Autodesk Inventor part; units mm, degrees
ref_plane "YZ Plane" through (0, 0, 0) normal (1, 0, 0) x (0, 1, 0)
ref_plane "XZ Plane" through (0, 0, 0) normal (0, 1, 0) x (-1, 0, 0)
ref_plane "XY Plane" through (0, 0, 0) normal (0, 0, 1) x (1, 0, 0)
sketch "Sketch1" plane through (0, 0, 0) normal (0, 1, 0) x (-1, 0, 0)
  circle A0 centre (0, 0) radius 2.4765
  circle A1 centre (-8.1903, -11.4773) radius 6 construction
  circle A2 centre (0, -14.1) radius 6 construction
  line L0 (0, -14.1) -> (-8.1903, -11.4773) construction
  circle A3 centre (-8.1903, -11.4773) radius 5.3 construction
  circle A4 centre (0, -14.1) radius 5.3 construction
  line L1 (-4.7712, -16.4078) -> (-5.6471, -16.1273)
  circle A5 centre (0, 0) radius 12.5 construction
  line L2 (-8.1903, -11.4773) -> (0, 0) construction
  arc A6 (-4.7712, -16.4078) -> (-2.2465, -12.2965) centre (-8.1903, -11.4773) ccw
  arc A7 (-5.3141, -11.3142) -> (-5.6471, -16.1273) centre (0, -14.1) ccw
  line L3 (2.3149, -16.9299) -> (1.4006, -17.0299)
  arc A8 (2.3149, -16.9299) -> (2.9491, -12.1471) centre (-2.814, -13.8163) ccw
  arc A9 (-0.2527, -12.4974) -> (1.4006, -17.0299) centre (5.735, -12.881) ccw
  line L4 (9.0008, -14.5246) -> (8.2062, -14.9879)
  arc A10 (9.0008, -14.5246) -> (7.6348, -9.8974) centre (3.0489, -13.7664) ccw
  arc A11 (4.8523, -11.5198) -> (8.2062, -14.9879) centre (10.4783, -9.4347) ccw
  line L5 (14.1303, -9.6079) -> (13.5929, -10.3543)
  arc A12 (14.1303, -9.6079) -> (11.0004, -5.9364) centre (8.3846, -11.3361) ccw
  arc A13 (9.1183, -8.5502) -> (13.5929, -10.3543) centre (13.4099, -4.3571) ccw
  line L6 (16.8166, -3.03) -> (16.6292, -3.9304)
  arc A14 (16.8166, -3.03) -> (12.4639, -0.9489) centre (12.2706, -6.9458) ccw
  arc A15 (11.8077, -4.1023) -> (16.6292, -3.9304) centre (14.0228, 1.4739) ccw
  line L7 (16.5951, 4.0719) -> (16.7902, 3.1731)
  arc A16 (16.5951, 4.0719) -> (11.7723, 4.2027) centre (14.0348, -1.3544) ccw
  arc A17 (12.4554, 1.055) -> (16.7902, 3.1731) centre (12.211, 7.05) ccw
  line L8 (13.5042, 10.4697) -> (14.048, 9.7279)
  arc A18 (13.5042, 10.4697) -> (9.0451, 8.6276) centre (13.3723, 4.4712) ccw
  arc A19 (10.9495, 6.0298) -> (14.048, 9.7279) centre (8.2878, 11.4071) ccw
  line L9 (8.0783, 15.0572) -> (8.8768, 14.6007)
  arc A20 (8.0783, 15.0572) -> (4.754, 11.5607) centre (10.3976, 9.5236) ccw
  arc A21 (7.5503, 9.9621) -> (8.8768, 14.6007) centre (2.9316, 13.7919) ccw
  line L10 (1.2556, 17.0412) -> (2.1707, 16.949)
  arc A22 (1.2556, 17.0412) -> (-0.3592, 12.4948) centre (5.6251, 12.9294) ccw
  arc A23 (2.8456, 12.1718) -> (2.1707, 16.949) centre (-2.9316, 13.7919) ccw
  line L11 (-5.7843, 16.0786) -> (-4.9107, 16.3665)
  arc A24 (-5.7843, 16.0786) -> (-5.4102, 11.2685) centre (-0.1201, 14.0995) ccw
  arc A25 (-2.3511, 12.2769) -> (-4.9107, 16.3665) centre (-8.2878, 11.4071) ccw
  line L12 (-11.824, 12.3359) -> (-11.1431, 12.9542)
  arc A26 (-11.824, 12.3359) -> (-9.5258, 8.0938) centre (-5.8445, 12.8317) ccw
  arc A27 (-7.1413, 10.2592) -> (-11.1431, 12.9542) centre (-12.211, 7.05) ccw
  line L13 (-15.8192, 6.4601) -> (-15.4486, 7.302)
  arc A28 (-15.8192, 6.4601) -> (-11.9943, 3.5195) centre (-10.5583, 9.3452) ccw
  arc A29 (-10.6967, 6.4676) -> (-15.4486, 7.302) centre (-14.0228, 1.4739) ccw
  line L14 (-17.0791, -0.5326) -> (-17.083, 0.3871)
  arc A30 (-17.0791, -0.5326) -> (-12.3888, -1.6633) centre (-13.4465, 4.2428) ccw
  arc A31 (-12.4026, 1.5577) -> (-17.083, 0.3871) centre (-13.4099, -4.3571) ccw
  line L15 (-15.3859, -7.4333) -> (-15.7636, -6.5946)
  arc A32 (-15.3859, -7.4333) -> (-10.6413, -6.5585) centre (-14.0097, -1.5932) ccw
  arc A33 (-11.9639, -3.6216) -> (-15.7636, -6.5946) centre (-10.4783, -9.4347) ccw
  arc A34 (-2.2465, -12.2965) -> (-0.2527, -12.4974) centre (0, 0) ccw
  arc A35 (2.9491, -12.1471) -> (4.8523, -11.5198) centre (0, 0) ccw
  arc A36 (7.6348, -9.8974) -> (9.1183, -8.5502) centre (0, 0) ccw
  arc A37 (11.0004, -5.9364) -> (11.8077, -4.1023) centre (0, 0) ccw
  arc A38 (12.4639, -0.9489) -> (12.4554, 1.055) centre (0, 0) ccw
  arc A39 (11.7723, 4.2027) -> (10.9495, 6.0298) centre (0, 0) ccw
  arc A40 (9.0451, 8.6276) -> (7.5503, 9.9621) centre (0, 0) ccw
  arc A41 (4.754, 11.5607) -> (2.8456, 12.1718) centre (0, 0) ccw
  arc A42 (-0.3592, 12.4948) -> (-2.3511, 12.2769) centre (0, 0) ccw
  arc A43 (-5.4102, 11.2685) -> (-7.1413, 10.2592) centre (0, 0) ccw
  arc A44 (-9.5258, 8.0938) -> (-10.6967, 6.4676) centre (0, 0) ccw
  arc A45 (-11.9943, 3.5195) -> (-12.4026, 1.5577) centre (0, 0) ccw
  arc A46 (-12.3888, -1.6633) -> (-11.9639, -3.6216) centre (0, 0) ccw
  arc A47 (-10.6413, -6.5585) -> (-9.4565, -8.1746) centre (0, 0) ccw
  line L16 (-11.0323, -13.0486) -> (-11.7185, -12.4361)
  arc A48 (-11.0323, -13.0486) -> (-7.0537, -10.3196) centre (-12.1505, -7.1537) ccw
  arc A49 (-9.4565, -8.1746) -> (-11.7185, -12.4361) centre (-5.735, -12.881) ccw
  arc A50 (-7.0537, -10.3196) -> (-5.3141, -11.3142) centre (0, 0) ccw
  point P0 (4.8523, -11.5198)
  point P1 (9.1183, -8.5502)
  point P2 (11.8077, -4.1023)
  point P3 (12.4554, 1.055)
  point P4 (10.9495, 6.0298)
  point P5 (7.5503, 9.9621)
  point P6 (2.8456, 12.1718)
  point P7 (-2.3511, 12.2769)
  point P8 (-7.1413, 10.2592)
  point P9 (-10.6967, 6.4676)
  point P10 (-12.4026, 1.5577)
  point P11 (-11.9639, -3.6216)
  point P12 (-9.4565, -8.1746)
  point P13 (-2.2465, -12.2965)
  point P14 (-0.2527, -12.4974)
  point P15 (2.9491, -12.1471)
  point P16 (4.8523, -11.5198)
  point P17 (7.6348, -9.8974)
  point P18 (9.1183, -8.5502)
  point P19 (11.0004, -5.9364)
  point P20 (11.8077, -4.1023)
  point P21 (12.4639, -0.9489)
  point P22 (12.4554, 1.055)
  point P23 (11.7723, 4.2027)
  point P24 (10.9495, 6.0298)
  point P25 (9.0451, 8.6276)
  point P26 (7.5503, 9.9621)
  point P27 (4.754, 11.5607)
  point P28 (2.8456, 12.1718)
  point P29 (-0.3592, 12.4948)
  point P30 (-2.3511, 12.2769)
  point P31 (-5.4102, 11.2685)
  point P32 (-7.1413, 10.2592)
  point P33 (-9.5258, 8.0938)
  point P34 (-10.6967, 6.4676)
  point P35 (-11.9943, 3.5195)
  point P36 (-12.4026, 1.5577)
  point P37 (-12.3888, -1.6633)
  point P38 (-11.9639, -3.6216)
  point P39 (-10.6413, -6.5585)
  point P40 (-5.3141, -11.3142)
  point P41 (-9.4565, -8.1746)
  point P42 (-7.0537, -10.3196)
  dimension "d3" = 10.6
  dimension "d0" = 4.953
  dimension "d1" = 12
  dimension "d2" = 8.6
  dimension "d4" = 25
  dimension "d5" = 14.1
  dimension "d6" = 14.1
  dimension "d9" = 360
  dimension "d13" = 360
extrude "Extrusion1" add sketch "Sketch1" along normal blind 6
properties part number "Gear_3DPrint"
For this review, take the finished solid that the model builds, in its own axes (mm). A direction names the side the tool comes from. Round coordinates to 2 decimals unless told otherwise and drop trailing zeros. Write each loop counter-clockwise with the first axis right and the second up, starting at its lowest first coordinate (ties: lowest second). Pieces come first, ordered by that corner, then holes. Notation, with made-up numbers: (70.25, -1) -> (95.25, -1) arc R18 ccw to (95.25, 11) -> close; hole circle Ø1 at (10.5, -21). An arc over 180 degrees is marked (long way). One line per question, with ' | ' between items. Start each with the question number.
(1) Tool access review of faces 5 (the face through (-12.93, 2.96, -7.42)), 6 (the face through (14.819, 2.958, -1.598)), 7 (the face through (11.1, 2.96, 9.94)): name each direction out of +Z, -Z, +X, -X, +Y, -Y from which nothing blocks a thin tool from reaching the whole face with its end or side.
(2) For line 1 along Z through (x, y) = (12.5, 3.75); line 2 along Z through (x, y) = (10.5, 0.35); line 3 along X through (y, z) = (4.4, 13.5), list the stretches that pass through material, from the lowest coordinate up. Write a range as from..to.
(3) Mouldability with a two-part tool opening along Z and no side actions: class faces 1 (the face through (10.073, 2.958, -7.402)), 2 (the face through (-11.049, 2.958, 10.003)), 3 (the face through (-1.86, 2.96, -16.98)), 4 (the face through (-8.793, 2.958, -12.034)) as released by +Z, released by -Z, zero draft, split by the parting line, or undercut.
(4) Add section B-B, the plane z = -7. Write out the cut boundary in (x, y), plus the area to 3 significant figures.
(5) Add section C-C, the plane z = 5.5. Write out the cut boundary in (x, y), plus the area to 3 significant figures.
(6) Insertion check: P1, Ø1.5, axis at y = 5, z = 1, coming from the -X side. The pin has a flat end and moves straight along its axis. Give the tip position at first contact, or say it passes through.
(7) Add section A-A, the plane x = 10. Write out the cut boundary in (y, z).
Answer list:
1) face 5: -X, +Y, -Y | face 6: +Y, -Y | face 7: +X, +Y, -Y
2) line 1: -7.4..-3.79, -1.68..1.57, 3.67..7.28 | line 2: -12.92..-9.23, -6.78..6.78, 9.05..12.8 | line 3: -8.92..-5.9, -3.06..0.35, 2.66..6.09
3) face 1: undercut | face 2: released by +Z | face 3: released by -Z | face 4: undercut
4) outline: (-12.53, 0) -> (10.36, 0) -> (10.36, 6) -> (-12.53, 6) -> close; (11.41, 0) -> (15.58, 0) -> (15.58, 6) -> (11.41, 6) -> close | area: 162 mm²
5) outline: (-11.22, 0) -> (15.16, 0) -> (15.16, 6) -> (-11.22, 6) -> close | area: 158 mm²
6) P1: x = -15.02
7) outline: (0, -12.76) -> (6, -12.76) -> (6, -8.66) -> (0, -8.66) -> close; (0, -7.5) -> (6, -7.5) -> (6, 7.5) -> (0, 7.5) -> close; (0, 8.5) -> (6, 8.5) -> (6, 12.63) -> (0, 12.63) -> close
